```python
from build123d import *

# Parameters (mm, degrees)
BOSS_EXTRUDE1_DEPTH = 6
FILLET1_R           = 1
SKETCH2_W           = 6
SKETCH2_H           = 20
CUT_EXTRUDE1_DEPTH  = 117.773284616


with BuildPart() as part:
    # Sketch1 → Boss-Extrude1 (new body)
    with BuildSketch(Plane.XY):
        Polygon((-10, 0), (10, 0), (10, 6), (60, 6), (60, 94), (10, 94), (10, 100), (-10, 100), (-10, 94), (-60, 94), (-60, 6), (-10, 6), align=None)
    extrude(amount=BOSS_EXTRUDE1_DEPTH)

    # Fillet1
    fillet1_edges = [part.edges().sort_by_distance(p)[0] for p in [
        (60, 94, 3),
        (60, 6, 3),
        (10, 6, 3),
        (10, 0, 3),
        (-10, 0, 3),
        (-10, 6, 3),
        (-60, 6, 3),
        (-60, 94, 3),
        (-10, 94, 3),
        (-10, 100, 3),
        (10, 100, 3),
        (10, 94, 3),
    ]]
    fillet(fillet1_edges, radius=FILLET1_R)

    # Sketch2 → Cut-Extrude1 (cut, through all)
    with BuildSketch(Plane(origin=(0, 0, 0), x_dir=(-1, 0, 0), z_dir=(0, 0, -1))):
        with Locations((57, 50)):
            Rectangle(SKETCH2_W, SKETCH2_H)
    extrude(amount=-CUT_EXTRUDE1_DEPTH, mode=Mode.SUBTRACT)


solid = part.part
```
Here's how the part is built. I have some questions about the finished solid (model axes, mm). A direction names the side the tool comes from. Give positions to 0.01 mm unless a question says otherwise; leave off trailing zeros. Order: outer loops, then holes, each group sorted by start corner. A loop starts at its lowest first (then second) coordinate and runs counter-clockwise, first axis right, second up. Notation, with made-up numbers: (82, 21) - (109, 21) arc R18 cw to (109, 26) - close; hole circle Ø7 at (48.5, 55.25). An arc over 180 degrees is marked (long way). Answer as a JSON object with one key per item and string values. Group by question number.
Item 1: If we section it at A-A on z = 2.55: Please give me the cut outline in (x, y), and give its area (3 significant figures).
Item 2: For P1, Ø1.8, axis at x = -29.5, z = 4, coming from the +Y side; P2, Ø1, axis at x = -37, z = 2.5, coming from the -Y side; P3, Ø1.2, axis at y = 96.5, z = 4, coming from the +X side, each with a flat end and sliding along its axis, tell me the tip position at first contact or that it passes through.
Item 3: If we section it at B-B on x = -43.5: Please give me the cut outline in (y, z), and give its area (3 significant figures).
Item 4: If we section it at C-C on y = 42: Please give me the cut outline in (x, z), and give its area (3 significant figures).
Item 5: If we mould it in two halves opening along Y, with no side actions, what happens to faces 1 (the flat face through (35, 94, 3)), 2 (the flat face through (-10, 3, 3)), 3 (the flat face through (-57, 40, 3))? For each: pulls with the +Y half, pulls with the -Y half, needs draft (parallel to the pull), parting line crosses it, or undercut.
Item 6: Which directions (+Z, -Z, +X, -X, +Y, -Y) give clear straight access to the entire face, cutting with the end or side of a thin tool? Please do faces 4 (the flat face through (-35, 94, 3)), 5 (the flat face through (10, 3, 3)), 6 (the flat face through (10, 97, 3)).
Item 7: Please list where these lines run through material, in increasing order: probe 1 along Y at (x, z) = (24.5, 3.5); probe 2 along X at (y, z) = (51.5, 2.7).
Result set:
{
 "1": {"outline": "(-60, 7) arc R1 ccw to (-59, 6) - (-11, 6) arc R1 cw to (-10, 5) - (-10, 1) arc R1 ccw to (-9, 0) - (9, 0) arc R1 ccw to (10, 1) - (10, 5) arc R1 cw to (11, 6) - (59, 6) arc R1 ccw to (60, 7) - (60, 93) arc R1 ccw to (59, 94) - (11, 94) arc R1 cw to (10, 95) - (10, 99) arc R1 ccw to (9, 100) - (-9, 100) arc R1 ccw to (-10, 99) - (-10, 95) arc R1 cw to (-11, 94) - (-59, 94) arc R1 ccw to (-60, 93) - (-60, 60) - (-54, 60) - (-54, 40) - (-60, 40) - close", "area": "10,700 mm²"},
 "2": {"P1": "y = 94", "P2": "y = 6", "P3": "x = 10"},
 "3": {"outline": "(6, 0) - (94, 0) - (94, 6) - (6, 6) - close", "area": "528 mm²"},
 "4": {"outline": "(-54, 0) - (60, 0) - (60, 6) - (-54, 6) - close", "area": "684 mm²"},
 "5": {"face 1": "pulls with the +Y half", "face 2": "needs draft", "face 3": "undercut"},
 "6": {"face 4": "+Z, -Z, -X, +Y", "face 5": "+Z, -Z, +X, -Y", "face 6": "+Z, -Z, +X, +Y"},
 "7": {"probe 1": "6 to 94", "probe 2": "-54 to 60"}
}
